The model under review builds one solid part; all positions refer to its coordinate system, in mm. Face numbers are marked on the shaded views. A direction names the side the tool comes from. Give positions to 0.01 mm unless a question says otherwise; leave off trailing zeros. Write each loop counter-clockwise with the first axis right and the second up, starting at its lowest first coordinate (ties: lowest second). Pieces come first, ordered by that corner, then holes. Notation, with made-up numbers: (0.25, 0) -> (29.25, 0) arc R23 ccw to (29.25, 24) -> close; hole circle Ø4 at (60.5, -12). An arc over 180 degrees is marked (long way). Use CSV: the item, a comma, the result in double quotes.
```python
from build123d import *

# Parameters (mm, degrees)
SKETCH1_R                = 15.5
BOSS_EXTRUDE1_DEPTH      = 57
SKETCH2_R                = 6
BOSS_EXTRUDE2_DEPTH      = 2.6
SKETCH3_W                = 58
SKETCH3_H                = 40
SKETCH3_R                = 2
SKETCH3_R_2              = 4
BOSS_EXTRUDE3_DEPTH      = 22.15
BOSS_EXTRUDE3_DEPTH_BACK = 13.75
FILLET1_R                = 1


with BuildPart() as part:
    # Sketch1 → Boss-Extrude1 (new body)
    with BuildSketch(Plane(origin=(0, 0, 0), x_dir=(0, 0, -1), z_dir=(1, 0, 0))):
        Circle(SKETCH1_R)
    extrude(amount=BOSS_EXTRUDE1_DEPTH)

    # Sketch2 → Boss-Extrude2 (add)
    with BuildSketch(Plane(origin=(57, 0, 0), x_dir=(0, 0, -1), z_dir=(1, 0, 0))):
        Circle(SKETCH2_R)
    extrude(amount=BOSS_EXTRUDE2_DEPTH)

    # Sketch3 → Boss-Extrude3 (add, two sides)
    with BuildSketch(Plane.XY) as boss_extrude3_sk:
        with Locations((-29, 0)):
            Rectangle(SKETCH3_W, SKETCH3_H)
        with Locations((-9, 13.75)):
            Circle(SKETCH3_R, mode=Mode.SUBTRACT)
        with Locations((-49.45, 13.75)):
            Circle(SKETCH3_R, mode=Mode.SUBTRACT)
        with Locations((-49.45, -13.75)):
            Circle(SKETCH3_R, mode=Mode.SUBTRACT)
        with Locations((-9, -13.75)):
            Circle(SKETCH3_R, mode=Mode.SUBTRACT)
        with Locations((-38, 0)):
            Circle(SKETCH3_R_2, mode=Mode.SUBTRACT)
    extrude(amount=BOSS_EXTRUDE3_DEPTH)
    extrude(boss_extrude3_sk.sketch, amount=-BOSS_EXTRUDE3_DEPTH_BACK)

    # Fillet1
    fillet1_edges = [part.edges().sort_by_distance(p)[0] for p in [
        (0, 20, 4.2),
        (0, -20, 4.2),
        (-58, -20, 4.2),
        (-58, 20, 4.2),
    ]]
    fillet(fillet1_edges, radius=FILLET1_R)


solid = part.part
```
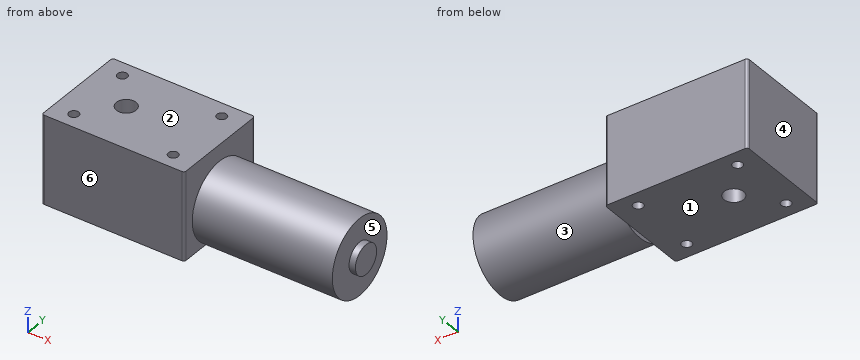
Q1. Consider section B-B (x = -38). Write out the cut boundary in (y, z), then the cut area to 3 significant figures.
Derived:
outline,"(-20, -13.75) -> (-4, -13.75) -> (-4, 22.15) -> (-20, 22.15) -> close; (4, -13.75) -> (20, -13.75) -> (20, 22.15) -> (4, 22.15) -> close"
area,"1,150 mm2"
Q2. Machinability: for the marked faces 5 and 6, which of the approach directions +Z, -Z, +X, -X, +Y, -Y give a long, thin tool a straight path to every point of the face, cutting with its end or side? Answer none if there is none.
Derived:
face 5,"+X"
face 6,"+Z, -Z, +X, -X, -Y"
Q3. To check wall thickness, follow probe 1 along X at (y, z) = (-14, 10.5); probe 2 along Y at (x, z) = (-9, 11.5); probe 3 along Z at (x, y) = (18, 0.5). State the ranges of each line that lie inside material, in increasing order.
Derived:
probe 1,"x = -58 to -51.43, -47.47 to -10.98, -7.02 to 0"
probe 2,"y = -20 to -15.75, -11.75 to 11.75, 15.75 to 20"
probe 3,"z = -15.49 to 15.49"
Q4. Consider section C-C (y = 13.75). Write out the cut boundary in (x, z).
Derived:
outline,"(-58, -13.75) -> (-51.45, -13.75) -> (-51.45, 22.15) -> (-58, 22.15) -> close; (-47.45, -13.75) -> (-11, -13.75) -> (-11, 22.15) -> (-47.45, 22.15) -> close; (-7, -13.75) -> (0, -13.75) -> (0, -7.15) -> (57, -7.15) -> (57, 7.15) -> (0, 7.15) -> (0, 22.15) -> (-7, 22.15) -> close"
Q5. Consider section A-A (y = 0). Write out the cut boundary in (x, z), then the cut area to 3 significant figures.
Derived:
outline,"(-58, -13.75) -> (-42, -13.75) -> (-42, 22.15) -> (-58, 22.15) -> close; (-34, -13.75) -> (0, -13.75) -> (0, -15.5) -> (57, -15.5) -> (57, -6) -> (59.6, -6) -> (59.6, 6) -> (57, 6) -> (57, 15.5) -> (0, 15.5) -> (0, 22.15) -> (-34, 22.15) -> close"
area,"3,590 mm2"
Q6. The part is to be moulded in two halves that separate along Z. For the marked faces 1, 2, 3 and 4, say which applies: pulls with the +Z half, pulls with the -Z half, needs draft (parallel to the pull), parting line crosses it, or undercut.
Derived:
face 1,"pulls with the -Z half"
face 2,"pulls with the +Z half"
face 3,"parting line crosses it"
face 4,"needs draft"
Q7. Consider section D-D (z = 18). Write out the cut boundary in (x, y).
Derived:
outline,"(-58, -19) arc R1 ccw to (-57, -20) -> (-1, -20) arc R1 ccw to (0, -19) -> (0, 19) arc R1 ccw to (-1, 20) -> (-57, 20) arc R1 ccw to (-58, 19) -> close; hole circle Ø4 at (-49.45, -13.75); hole circle Ø4 at (-49.45, 13.75); hole circle Ø8 at (-38, 0); hole circle Ø4 at (-9, -13.75); hole circle Ø4 at (-9, 13.75)"
Q8. Insertion check: pin 1 (1 mm diameter, centred on y = -1.5, z = 16, fed in from +X); pin 2 (4 mm diameter, centred on x = 6, y = 7, fed in from +Z); pin 3 (4 mm diameter, centred on y = 3.5, z = 10.5, fed in from +X). Each pin has a flat end and moves straight along its axis. Give the tip position at first contact, or say it passes through.
Derived:
pin 1,"stops at x = 0"
pin 2,"stops at z = 14.67"
pin 3,"stops at x = 57"
